from build123d import *

# Parameters (mm, degrees)
SKETCH1_W                       = 30
SKETCH1_H                       = 80
BOSS_EXTRUDE1_DEPTH             = 3
BOSS_EXTRUDE2_DEPTH             = 3
SKETCH3_R                       = 5
CUT_EXTRUDE1_DEPTH              = 86.492689746
CHAMFER1_SIZE                   = 2
SKETCH4_R                       = 1.5
CUT_EXTRUDE2_DEPTH              = 86.650452421
SKETCH5_W                       = 10
SKETCH5_H                       = 3
BOSS_EXTRUDE3_DEPTH             = 10
F_3_0MM_DOWEL_HOLE1_D           = 3
F_3_0MM_DOWEL_HOLE1_CSINK_D     = 3.05
F_3_0MM_DOWEL_HOLE1_CSINK_ANGLE = 90


with BuildPart() as part:
    # Sketch1 → Boss-Extrude1 (new body)
    with BuildSketch(Plane(origin=(0, 0, 0), x_dir=(1, 0, 0), z_dir=(0, 1, 0))):
        with Locations((15, 40)):
            Rectangle(SKETCH1_W, SKETCH1_H)
    extrude(amount=BOSS_EXTRUDE1_DEPTH)

    # Sketch2 → Boss-Extrude2 (add)
    with BuildSketch(Plane(origin=(0, 3, 0), x_dir=(1, 0, 0), z_dir=(0, 1, 0))):
        with BuildLine():
            Line((15, 80), (0, 80))
            Line((0, 80), (0, 26.770509831))
            ThreePointArc((0, 26.770509831), (6.97150298, 31.018878077), (15, 32.5))
            Line((15, 32.5), (15, 80))
        make_face()
        with BuildLine():
            Line((30, 80), (15, 80))
            Line((15, 80), (15, 32.5))
            ThreePointArc((15, 32.5), (23.02849702, 31.018878077), (30, 26.770509831))
            Line((30, 26.770509831), (30, 80))
        make_face()
    extrude(amount=BOSS_EXTRUDE2_DEPTH)

    # Sketch3 → Cut-Extrude1 (cut, through all)
    with BuildSketch(Plane(origin=(0, 3, 0), x_dir=(1, 0, 0), z_dir=(0, 1, 0))):
        with Locations(Location((15, 10, 0), (0, 0, 270))):
            Circle(SKETCH3_R)
    extrude(amount=-CUT_EXTRUDE1_DEPTH, mode=Mode.SUBTRACT)

    # Chamfer1
    chamfer1_edges = [part.edges().sort_by_distance(p)[0] for p in [
        (0, 3, -80),
        (30, 3, -80),
        (30, 1.5, 0),
        (0, 1.5, 0),
    ]]
    chamfer(chamfer1_edges, length=CHAMFER1_SIZE)

    # Sketch4 → Cut-Extrude2 (cut, through all)
    with BuildSketch(Plane(origin=(0, 6, 0), x_dir=(1, 0, 0), z_dir=(0, 1, 0))):
        with Locations(Location((3.75, 65, 0), (0, 0, 270))):
            Circle(SKETCH4_R)
        with Locations(Location((26.25, 65, 0), (0, 0, 270))):
            Circle(SKETCH4_R)
    extrude(amount=-CUT_EXTRUDE2_DEPTH, mode=Mode.SUBTRACT)

    # Sketch5 → Boss-Extrude3 (add)
    with BuildSketch(Plane.ZY):
        with Locations((-35, 1.5)):
            Rectangle(SKETCH5_W, SKETCH5_H)
    boss_extrude3 = extrude(amount=BOSS_EXTRUDE3_DEPTH)

    # Ø3.0mm Dowel Hole1 (through all)
    with Locations(Plane(origin=(0, 6, 0), x_dir=(1, 0, 0), z_dir=(0, 1, 0))):
        with Locations((-5, 35)):
            f_3_0mm_dowel_hole1 = CounterSinkHole(F_3_0MM_DOWEL_HOLE1_D / 2, F_3_0MM_DOWEL_HOLE1_CSINK_D / 2, counter_sink_angle=F_3_0MM_DOWEL_HOLE1_CSINK_ANGLE)

    # Mirror1: Boss-Extrude3, Ø3.0mm Dowel Hole1 across plane
    add(boss_extrude3.mirror(Plane.ZY.offset(-15)))
    add(f_3_0mm_dowel_hole1.mirror(Plane.ZY.offset(-15)), mode=Mode.SUBTRACT)


solid = part.part
The model under review builds one solid part; all positions refer to its coordinate system, in mm. A direction names the side the tool comes from. Give positions to 0.01 mm unless a question says otherwise; leave off trailing zeros. Write each loop counter-clockwise with the first axis right and the second up, starting at its lowest first coordinate (ties: lowest second). Pieces come first, ordered by that corner, then holes.
1. For P1, Ø15, axis at x = 17, z = -24, coming from the +Y side; P2, Ø1.5, axis at x = -5, y = 1.5, coming from the +Z side; P3, Ø8, axis at x = 15, z = -10, coming from the +Y side; P4, Ø3.5, axis at x = 35.5, y = 1, coming from the -Z side, all flat-tipped, find the tip position at first contact; note any pin that passes through.
2. Add section B-B, the plane x = 35. Write out the cut boundary in (y, z), plus the area to 3 significant figures.
3. Wall thickness on L1, parallel to X at y = 0.3, z = -65; L2, parallel to Z at x = -5, y = 1.1; L3, parallel to X at y = 4.5, z = -48: over which ranges is each line inside the solid? List them lowest first.
4. Draft analysis for pull direction Z (two halves, no side actions). For faces 1 (the flat face through (1, 1, -1)), 2 (the flat face through (0, 3, -49)), 3 (the cylindrical face through (33.8, 1.5, -34.1)), 4 (the cylindrical face through (10.564, 1.521, -7.693)), state which applies: +Z half, -Z half, draft (parallel to the pull), parting line (faces both ways), or undercut.
5. Add section D-D, the plane y = 4.95. Write out the cut boundary in (x, z).
6. Add section A-A, the plane z = -35. Write out the cut boundary in (x, y), plus the area to 3 significant figures.
7. Add section C-C, the plane z = -10. Write out the cut boundary in (x, y).
8. Tool access review of faces 5 (the flat face through (-5, 1, -30)), 6 (the flat face through (33.8, 3, -36.2)), 7 (the flat face through (15, 3, -16)), 8 (the flat face through (35, 1, -30)): name each direction out of +Z, -Z, +X, -X, +Y, -Y from which nothing blocks a thin tool from reaching the whole face with its end or side.
Worked answers:
1. P1: stops at y = 3
1. P2: stops at z = -30
1. P3: passes through
1. P4: stops at z = -40
2. outline: (0, -40) - (3, -40) - (3, -36.5) - (0, -36.5) - close; (0, -33.5) - (3, -33.5) - (3, -30) - (0, -30) - close
2. area: 21.0 mm2
3. L1: x = 0 to 2.25, 5.25 to 24.75, 27.75 to 30
3. L2: z = -40 to -36.5, -33.5 to -30
3. L3: x = 0 to 30
4. face 1: +Z half
4. face 2: draft
4. face 3: undercut
4. face 4: undercut
5. outline: (0, -78) - (2, -80) - (28, -80) - (30, -78) - (30, -26.77) arc R22.5 cw to (0, -26.77) - close; hole circle Ø3 at (3.75, -65); hole circle Ø3 at (26.25, -65)
6. outline: (-10, 0) - (-6.5, 0) - (-6.5, 3) - (-10, 3) - close; (-3.5, 0) - (33.5, 0) - (33.5, 3) - (30, 3) - (30, 6) - (0, 6) - (0, 3) - (-3.5, 3) - close; (36.5, 0) - (40, 0) - (40, 3) - (36.5, 3) - close
6. area: 222 mm2
7. outline: (0, 0) - (10, 0) - (10, 3) - (0, 3) - close; (20, 0) - (30, 0) - (30, 3) - (20, 3) - close
8. face 5: +Z, -X, +Y, -Y
8. face 6: +Z, -Z, +X, +Y
8. face 7: +Z, +Y
8. face 8: +Z, +X, +Y, -Y
